Answer from the drawing. Dimensions are ordinates in mm from the lowest x, y and z of the part. A direction names the side the tool comes from. Give positions to 0.01 mm unless a question says otherwise; leave off trailing zeros. Write each loop counter-clockwise with the first axis right and the second up, starting at its lowest first coordinate (ties: lowest second). Pieces come first, ordered by that corner, then holes.
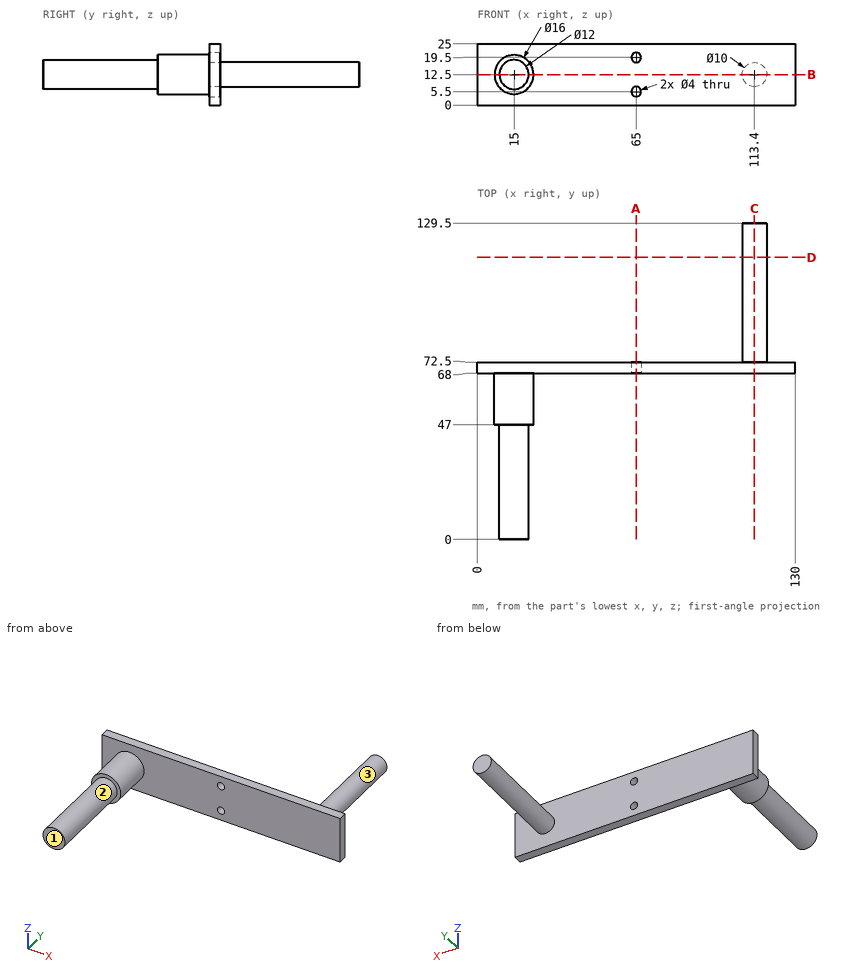
Item 1: Section A-A (x = 65) is taken. Write down the section's boundary in (y, z), and give its area (3 significant figures).
Result set:
outline: (68, 0) - (72.5, 0) - (72.5, 3.5) - (68, 3.5) - close; (68, 7.5) - (72.5, 7.5) - (72.5, 17.5) - (68, 17.5) - close; (68, 21.5) - (72.5, 21.5) - (72.5, 25) - (68, 25) - close
area: 76.5 mm2
Item 2: Section B-B (z = 12.5) is taken. Write down the section's boundary in (x, y), and give its area (4 significant figures).
Result set:
outline: (0, 68) - (7, 68) - (7, 47) - (9, 47) - (9, 0) - (21, 0) - (21, 47) - (23, 47) - (23, 68) - (130, 68) - (130, 72.5) - (118.4, 72.5) - (118.4, 129.5) - (108.4, 129.5) - (108.4, 72.5) - (0, 72.5) - close
area: 2,055 mm2
Item 3: Section C-C (x = 113.4) is taken. Write down the section's boundary in (y, z), and give its area (4 significant figures).
Result set:
outline: (68, 0) - (72.5, 0) - (72.5, 7.5) - (129.5, 7.5) - (129.5, 17.5) - (72.5, 17.5) - (72.5, 25) - (68, 25) - close
area: 682.5 mm2
Item 4: Each of these flat-tipped pins is pushed along its axis until it touches: pin 1 Ø6.5 at (x, z) = (65, 5.5) entering from +Y; pin 2 Ø3 at (x, z) = (96.5, 6) entering from -Y; pin 3 Ø13 at (x, z) = (11.5, 10.5) entering from -Y; pin 4 Ø1 at (y, z) = (112, 7.5) entering from +X. Where does it stop, or does it pass through?
Result set:
pin 1: stops at y = 72.5
pin 2: stops at y = 68
pin 3: stops at y = 0
pin 4: stops at x = 115.58
Item 5: Section D-D (y = 115.5) is taken. Write down the section's boundary in (x, z).
Result set:
outline: circle Ø10 at (113.4, 12.5)
Item 6: Find the intervals of material crossed by line 1 along X through (y, z) = (70.4, 5.5); line 2 along Y through (x, z) = (29.5, 10.75); line 3 along Y through (x, z) = (115.5, 8.75), in increasing order.
Result set:
line 1: x = 0 to 63, 67 to 130
line 2: y = 68 to 72.5
line 3: y = 68 to 129.5
Item 7: Which of the six approach directions +Z, -Z, +X, -X, +Y, -Y give full straight-line access (tool end or side, diameter ignored) to the marked faces 1, 2 and 3?
Result set:
face 1: +Z, -Z, +X, -X, -Y
face 2: -Y
face 3: +Y
